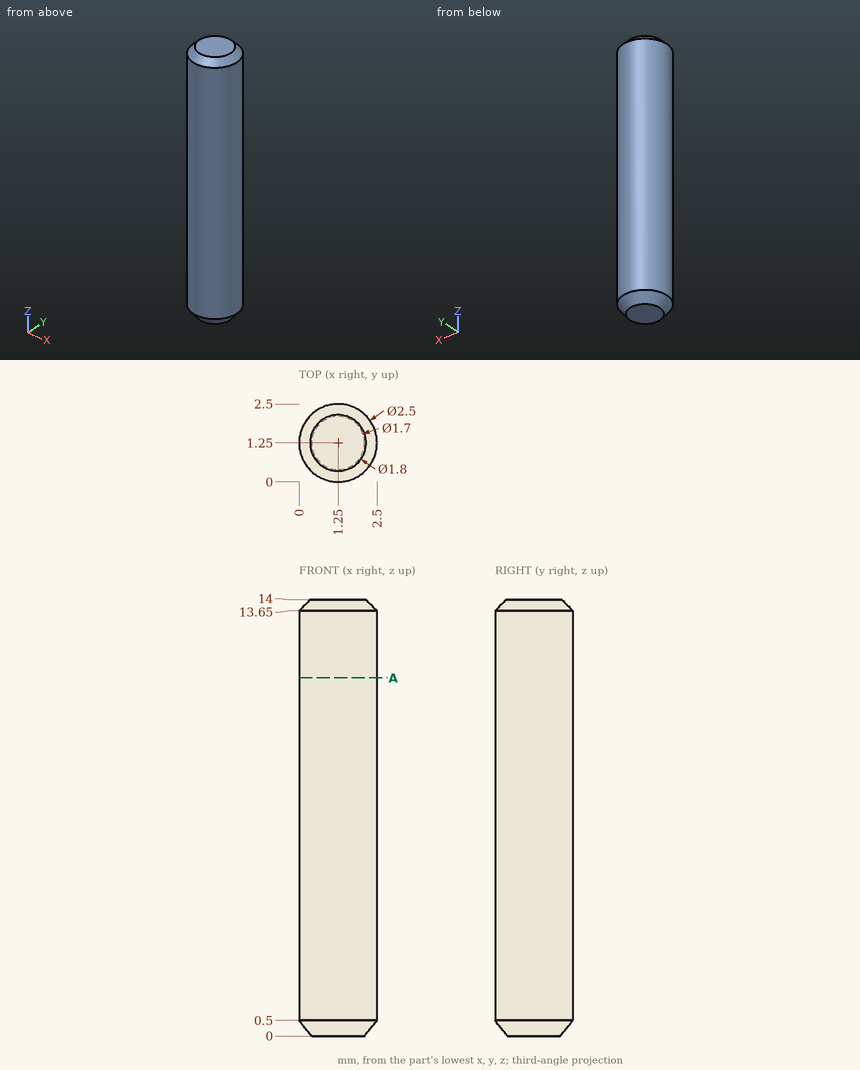
Input: dimensioned drawing with shaded views. Units: mm. Origin: part minimum x, y, z. Round coordinates to 2 decimals unless told otherwise and drop trailing zeros. Loops run counter-clockwise (first coordinate to the right, second up) from the corner with the lowest first, then second, coordinate; pieces in that order, holes last. Notation, with made-up numbers: (-15.75, -36.5) -> (8.25, -36.5) arc R7 ccw to (8.25, -24.5) -> close; hole circle Ø7 at (-3, 51). An arc over 180 degrees is marked (long way). Use one line per item in the form item = value. Start each with the question number.
1) Section A-A on z = 11.5. Output: boundary loops of the cut face in (x, y).
2) Line query: L1, parallel to X at y = 1.2, z = 2.75; L2, parallel to X at y = 1.95, z = 11.75. Output: solid intervals per line, ascending.
3) First-contact query: P1, Ø1, axis at y = 2, z = 2.5, coming from the +X side; P2, Ø1, axis at y = 2, z = 9.5, coming from the -X side. Flat tips, straight axial feed; report the tip coordinate or a pass-through.
Response:
q1.outline = circle Ø2.5 at (1.25, 1.25)
q2.L1 = 0 to 2.5
q2.L2 = 0.21 to 2.29
q3.P1 = 2.47
q3.P2 = 0.03
